```python
from build123d import *

# Parameters (mm, degrees)
MODEL_W             = 5.5
MODEL_H             = 5.5
BOSS_EXTRUDE1_DEPTH = 6


with BuildPart() as part:
    # Model → Boss-Extrude1 (new body)
    with BuildSketch(Plane.XY):
        with BuildLine():
            Line((3452.90039403, 1295.068502361), (3452.90039403, 1271.068502361))
            Line((3452.90039403, 1271.068502361), (3462.90039403, 1271.068502361))
            Line((3462.90039403, 1271.068502361), (3473.90039403, 1271.068502361))
            Line((3473.90039403, 1271.068502361), (3473.90039403, 1302.068502361))
            Line((3473.90039403, 1302.068502361), (3463.502374277, 1302.068502361))
            ThreePointArc((3463.502374277, 1302.068502361), (3503.90039403, 1336.068502361), (3544.298413784, 1302.068502361))
            Line((3544.298413784, 1302.068502361), (3533.90039403, 1302.068502361))
            Line((3533.90039403, 1302.068502361), (3533.90039403, 1271.068502361))
            Line((3533.90039403, 1271.068502361), (3536.40039403, 1271.068502361))
            Line((3536.40039403, 1271.068502361), (3536.40039403, 1265.068502361))
            Line((3536.40039403, 1265.068502361), (3542.40039403, 1265.068502361))
            Line((3542.40039403, 1265.068502361), (3542.40039403, 1271.068502361))
            Line((3542.40039403, 1271.068502361), (3554.90039403, 1271.068502361))
            Line((3554.90039403, 1271.068502361), (3554.90039403, 1295.068502361))
            ThreePointArc((3554.90039403, 1295.068502361), (3503.90039403, 1346.068502361), (3452.90039403, 1295.068502361))
        make_face()
        with Locations((3539.40039403, 1276.568502361)):
            Rectangle(MODEL_W, MODEL_H, mode=Mode.SUBTRACT)
        with Locations((3539.40039403, 1296.568502361)):
            Rectangle(MODEL_W, MODEL_H, mode=Mode.SUBTRACT)
        with Locations((3468.40039403, 1276.568502361)):
            Rectangle(MODEL_W, MODEL_H, mode=Mode.SUBTRACT)
        with Locations((3468.40039403, 1296.568502361)):
            Rectangle(MODEL_W, MODEL_H, mode=Mode.SUBTRACT)
    extrude(amount=BOSS_EXTRUDE1_DEPTH)


solid = part.part
```
Design review of the part built by this model. Coordinates are the model's own, in mm. A direction names the side the tool comes from. Give positions to 0.01 mm unless a question says otherwise; leave off trailing zeros. Write each loop counter-clockwise with the first axis right and the second up, starting at its lowest first coordinate (ties: lowest second). Pieces come first, ordered by that corner, then holes. Notation, with made-up numbers: (80, 60.5) - (104, 60.5) arc R26 ccw to (104, 74.5) - close; hole circle Ø10 at (24.25, 27). An arc over 180 degrees is marked (long way). Return JSON: item names as keys, results as strings. Group by question number.
(1) We need section A-A, the plane y = 1288. Give the boundary of the cut face in (x, z), then the cut area to 3 significant figures.
(2) Machinability: for faces 4 (the flat face through (3463, 1271.069, 3)), 5 (the flat face through (3542.4, 1268, 3)), 6 (the flat face through (3465.65, 1277, 3)), which of the approach directions +Z, -Z, +X, -X, +Y, -Y give a long, thin tool a straight path to every point of the face, cutting with its end or side? Answer none if there is none.
(3) We need section C-C, the plane z = 2.75. Give the number of separate pieces and of enclosed holes in the cut face, then the cut area to 3 significant figures.
(4) Mouldability with a two-part tool opening along X and no side actions: class faces 1 (the flat face through (3471.15, 1297, 3)), 2 (the flat face through (3536.4, 1268, 3)), 3 (the flat face through (3549, 1271.069, 3)) as +X half, -X half, draft (parallel to the pull), parting line (faces both ways), or undercut.
(5) We need section D-D, the plane y = 1317. Give the boundary of the cut face in (x, z).
(6) Insertion check: pin 1 (3 mm diameter, centred on x = 3468.5, z = 3, fed in from +Y); pin 2 (3 mm diameter, centred on x = 3547.5, z = 2, fed in from -Y); pin 3 (1.8 mm diameter, centred on y = 1269.5, z = 2.5, fed in from +X). Each pin has a flat end and moves straight along its axis. Give the tip position at first contact, or say it passes through.
(7) We need section B-B, the plane x = 3469. Give the boundary of the cut face in (y, z).
(8) To check wall thickness, follow probe 1 along X at (y, z) = (1275, 0.4); probe 2 along X at (y, z) = (1292, 2.55); probe 3 along X at (y, z) = (1298.5, 2.95). State the ranges of each line that lie inside material, in increasing order.
Reported:
{
 "1": {"outline": "(3452.9, 0) - (3473.9, 0) - (3473.9, 6) - (3452.9, 6) - close; (3533.9, 0) - (3554.9, 0) - (3554.9, 6) - (3533.9, 6) - close", "area": "252 mm2"},
 "2": {"face 4": "+Z, -Z, -X, -Y", "face 5": "+Z, -Z, +X, -Y", "face 6": "+Z, -Z"},
 "3": {"separate pieces": "1", "enclosed holes": "4", "area": "2,520 mm2"},
 "4": {"face 1": "undercut", "face 2": "-X half", "face 3": "draft"},
 "5": {"outline": "(3457.86, 0) - (3469.26, 0) - (3469.26, 6) - (3457.86, 6) - close; (3538.54, 0) - (3549.94, 0) - (3549.94, 6) - (3538.54, 6) - close"},
 "6": {"pin 1": "stops at y = 1333.17", "pin 2": "stops at y = 1271.07", "pin 3": "stops at x = 3542.4"},
 "7": {"outline": "(1271.07, 0) - (1273.82, 0) - (1273.82, 6) - (1271.07, 6) - close; (1279.32, 0) - (1293.82, 0) - (1293.82, 6) - (1279.32, 6) - close; (1299.32, 0) - (1302.07, 0) - (1302.07, 6) - (1299.32, 6) - close; (1316.59, 0) - (1332.26, 0) - (1332.26, 6) - (1316.59, 6) - close"},
 "8": {"probe 1": "x = 3452.9 to 3465.65, 3471.15 to 3473.9, 3533.9 to 3536.65, 3542.15 to 3554.9", "probe 2": "x = 3452.9 to 3473.9, 3533.9 to 3554.9", "probe 3": "x = 3453.02 to 3465.65, 3471.15 to 3473.9, 3533.9 to 3536.65, 3542.15 to 3554.78"}
}
